For this review, take the finished solid that the model builds, in its own axes (mm). A direction names the side the tool comes from. Coordinates: 2 decimals unless noted, no trailing zeros. Loops run counter-clockwise (first coordinate to the right, second up) from the corner with the lowest first, then second, coordinate; pieces in that order, holes last. Notation, with made-up numbers: (74.5, -30.5) - (105.5, -30.5) arc R35 ccw to (105.5, 5.5) - close; hole circle Ø4 at (59.25, 61). An arc over 180 degrees is marked (long way). Answer as a JSON object with one key per item and string values. Group by question number.
Item 1: To check wall thickness, follow line 1 (Y direction, x = 0, z = 9.5); line 2 (Z direction, x = 11, y = -3.5); line 3 (Z direction, x = 1, y = 3.5). State the ranges of each line that lie inside material, in increasing order.
Item 2: Clearance check with flat-ended pins moving along their axes: pin 1 (9 mm diameter, centred on x = 0, y = 0, fed in from +Z); pin 2 (1.5 mm diameter, centred on x = -11.5, z = 2, fed in from -Y); pin 3 (4 mm diameter, centred on x = 4.5, z = -4, fed in from +Y). State where each tip first meets the part, or that it passes through.
Item 3: Tool access review of faces 1 (the flat face through (6, 0, 12)), 2 (the cylindrical face through (-1.08, -4.88, 8.55)), 3 (the flat face through (-9, 8, 0)): name each direction out of +Z, -Z, +X, -X, +Y, -Y from which nothing blocks a thin tool from reaching the whole face with its end or side.
Item 4: Mouldability with a two-part tool opening along X and no side actions: class faces 4 (the flat face through (2.2, -3.3, 5)), 5 (the flat face through (0, 4, -8)), 6 (the cylindrical face through (-2.17, 9.76, -4.7)) as released by +X, released by -X, zero draft, split by the parting line, or undercut.
Item 5: We need section D-D (z = -2.75). Give the boundary of the cut face in (x, y), then the cut area to 3 significant figures.
Item 6: We need section A-A (y = 0). Give the boundary of the cut face in (x, z), then the cut area to 3 significant figures.
Item 7: We need section C-C (z = 9). Give the boundary of the cut face in (x, y).
from build123d import *

# Parameters (mm, degrees)
F0_R           = 16
F1_DEPTH       = 12
F2_R           = 10
F3_DEPTH       = 8
F5_D           = 7
F5_CBORE_D     = 10
F5_CBORE_DEPTH = 7
F6_R           = 1.5


with BuildPart() as f1:
    # F0 (on Top) → F1 (new body)
    with BuildSketch(Plane.XY):
        Circle(F0_R)
    extrude(amount=F1_DEPTH)

    # F2 (on face) → F3 (join)
    with BuildSketch(Plane(origin=(0, 0, 0), x_dir=(1, 0, 0), z_dir=(0, 0, -1))):
        Circle(F2_R)
    extrude(amount=F3_DEPTH)

    # F5 (through all)
    with Locations(Plane.XY.offset(12)):
        with Locations((0, 0)):
            CounterBoreHole(F5_D / 2, F5_CBORE_D / 2, F5_CBORE_DEPTH)

    # F6
    f6_edges = [f1.edges().sort_by_distance(p)[0] for p in [
        (-16, 0, 12),
        (-16, 0, 0),
        (-10, 0, 0),
    ]]
    fillet(f6_edges, radius=F6_R)


solid = f1.part
Check sheet entries:
{
 "1": {"line 1": "y = -16 to -5, 5 to 16", "line 2": "z = 0 to 12", "line 3": "z = -8 to 5"},
 "2": {"pin 1": "stops at z = 5", "pin 2": "stops at y = -11.85", "pin 3": "stops at y = 9.68"},
 "3": {"face 1": "+Z, +X, -X, +Y, -Y", "face 2": "+Z", "face 3": "-Z"},
 "4": {"face 4": "undercut", "face 5": "zero draft", "face 6": "split by the parting line"},
 "5": {"outline": "circle Ø20 at (0, 0); hole circle Ø7 at (0, 0)", "area": "276 mm2"},
 "6": {"outline": "(-16, 1.5) arc R1.5 ccw to (-14.5, 0) - (-11.5, 0) arc R1.5 cw to (-10, -1.5) - (-10, -8) - (-3.5, -8) - (-3.5, 5) - (-5, 5) - (-5, 12) - (-14.5, 12) arc R1.5 ccw to (-16, 10.5) - close; (3.5, -8) - (10, -8) - (10, -1.5) arc R1.5 cw to (11.5, 0) - (14.5, 0) arc R1.5 ccw to (16, 1.5) - (16, 10.5) arc R1.5 ccw to (14.5, 12) - (5, 12) - (5, 5) - (3.5, 5) - close", "area": "382 mm2"},
 "7": {"outline": "circle Ø32 at (0, 0); hole circle Ø10 at (0, 0)"}
}
